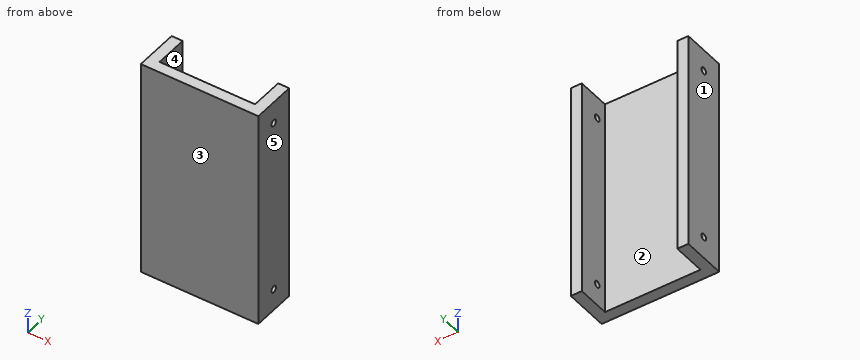
from build123d import *

# Parameters (mm, degrees)
ESQUISSE1_W             = 53.3
ESQUISSE1_H             = 100
BOSS_EXTRU_1_DEPTH      = 20
ESQUISSE2_W             = 43.3
ESQUISSE2_H             = 100
ENL_V_MAT_EXTRU_1_DEPTH = 15
ESQUISSE3_R             = 1.5
ENL_V_MAT_EXTRU_2_DEPTH = 54.3


with BuildPart() as part:
    # Esquisse1 → Boss.-Extru.1 (new body)
    with BuildSketch(Plane(origin=(0, 0, 0), x_dir=(1, 0, 0), z_dir=(0, 1, 0))):
        with Locations((26.65, -50)):
            Rectangle(ESQUISSE1_W, ESQUISSE1_H)
    extrude(amount=BOSS_EXTRU_1_DEPTH)

    # Esquisse2 → Enlèv. mat.-Extru.1 (cut)
    with BuildSketch(Plane(origin=(0, 20, 0), x_dir=(1, 0, 0), z_dir=(0, 1, 0))):
        with Locations((26.65, -50)):
            Rectangle(ESQUISSE2_W, ESQUISSE2_H)
    extrude(amount=-ENL_V_MAT_EXTRU_1_DEPTH, mode=Mode.SUBTRACT)

    # Esquisse3 → Enlèv. mat.-Extru.2 (cut, through all)
    with BuildSketch(Plane(origin=(53.3, 0, 0), x_dir=(0, 0, -1), z_dir=(1, 0, 0))):
        with Locations((-90, 10)):
            Circle(ESQUISSE3_R)
        with Locations((-10, 10)):
            Circle(ESQUISSE3_R)
    extrude(amount=-ENL_V_MAT_EXTRU_2_DEPTH, mode=Mode.SUBTRACT)


solid = part.part
Build history of the part. All positions in model axes, mm. Face numbers are marked on the shaded views. A direction names the side the tool comes from. Coordinates: 2 decimals unless noted, no trailing zeros. Write each loop counter-clockwise with the first axis right and the second up, starting at its lowest first coordinate (ties: lowest second). Pieces come first, ordered by that corner, then holes.
(1) Drill centre lines: line 1 (X direction, y = 13.5, z = 25); line 2 (Y direction, x = 2.3, z = 10); line 3 (Y direction, x = 34.5, z = 35.5). Where is each one in solid material? Low to high.
(2) Mould opens along X. For the marked faces 3, 4 and 5 say: pulls with the +X half, pulls with the -X half, needs draft (parallel to the pull), parting line crosses it, or undercut.
(3) Pin check, flat tips, straight feed: pin 1 Ø12 at (y, z) = (14.5, 40.5) entering from -X; pin 2 Ø2.5 at (y, z) = (10, 90) entering from +X; pin 3 Ø4 at (x, z) = (37, 72) entering from +Y. Stop position of each tip, or through.
(4) Cut at A-A on y = 10. List the corners of the cut face in (x, z), and give its area (3 significant figures).
(5) Cut at C-C on z = 55. List the corners of the cut face in (x, y), and give its area (4 significant figures).
(6) 3-axis set-ups, long thin cutter, end or side, ignore diameter. For the marked faces 1 and 2: which of +Z, -Z, +X, -X, +Y, -Y reach the whole face in a straight line?
(7) Cut at D-D on x = 7. List the corners of the cut face in (y, z).
(8) Cut at B-B on z = 90. List the corners of the cut face in (x, y).
Working result:
1. line 1: x = 0 to 5, 48.3 to 53.3
1. line 2: y = 0 to 8.5, 11.5 to 20
1. line 3: y = 0 to 5
2. face 3: needs draft
2. face 4: undercut
2. face 5: pulls with the +X half
3. pin 1: stops at x = 0
3. pin 2: passes through
3. pin 3: stops at y = 5
4. outline: (0, 0) - (5, 0) - (5, 8.5) - (0, 8.5) - close; (0, 11.5) - (5, 11.5) - (5, 88.5) - (0, 88.5) - close; (0, 91.5) - (5, 91.5) - (5, 100) - (0, 100) - close; (48.3, 0) - (53.3, 0) - (53.3, 8.5) - (48.3, 8.5) - close; (48.3, 11.5) - (53.3, 11.5) - (53.3, 88.5) - (48.3, 88.5) - close; (48.3, 91.5) - (53.3, 91.5) - (53.3, 100) - (48.3, 100) - close
4. area: 940 mm2
5. outline: (0, 0) - (53.3, 0) - (53.3, 20) - (48.3, 20) - (48.3, 5) - (5, 5) - (5, 20) - (0, 20) - close
5. area: 416.5 mm2
6. face 1: +Z, -Z, -X, +Y, -Y
6. face 2: +Z, -Z, +Y
7. outline: (0, 0) - (5, 0) - (5, 100) - (0, 100) - close
8. outline: (0, 0) - (53.3, 0) - (53.3, 8.5) - (48.3, 8.5) - (48.3, 5) - (5, 5) - (5, 8.5) - (0, 8.5) - close; (0, 11.5) - (5, 11.5) - (5, 20) - (0, 20) - close; (48.3, 11.5) - (53.3, 11.5) - (53.3, 20) - (48.3, 20) - close
